Could you check a few things on this model? Use its own coordinates, in mm. Give positions to 0.01 mm unless a question says otherwise; leave off trailing zeros. Write each loop counter-clockwise with the first axis right and the second up, starting at its lowest first coordinate (ties: lowest second). Pieces come first, ordered by that corner, then holes. Notation, with made-up numbers: (73.5, 54) - (96.5, 54) arc R20 cw to (96.5, 74) - close; hole circle Ø2 at (34.25, -1). An arc over 180 degrees is marked (long way). Use one line per item in the form item = value.
```python
from build123d import *

# Parameters (mm, degrees)
F0_R     = 2.0193
F0_R_2   = 14.2875
F0_R_3   = 2.5527
F0_R_4   = 2.8575
F1_DEPTH = 6.35


with BuildPart() as f1:
    # F0 (on Front) → F1 (new body)
    with BuildSketch(Plane.XZ):
        with BuildLine():
            ThreePointArc((-49.323942, 42.948766), (-63.830824, 30.807895), (-82.659198, 28.979589))
            ThreePointArc((-82.659198, 28.979589), (-86.073502, 27.415326), (-85.607225, 23.688803))
            Line((-85.607225, 23.688803), (-45.021703, -19.243367))
            ThreePointArc((-45.021703, -19.243367), (-41.868292, -21.447891), (-38.1, -22.225))
            Line((-38.1, -22.225), (38.1, -22.225))
            ThreePointArc((38.1, -22.225), (41.868292, -21.447891), (45.021703, -19.243367))
            Line((45.021703, -19.243367), (85.607225, 23.688803))
            ThreePointArc((85.607225, 23.688803), (86.073502, 27.415326), (82.659198, 28.979589))
            ThreePointArc((82.659198, 28.979589), (63.830824, 30.807895), (49.323942, 42.948766))
            Line((49.323942, 42.948766), (22.663343, 84.185078))
            ThreePointArc((22.663343, 84.185078), (0, 96.52), (-22.663343, 84.185078))
            Line((-22.663343, 84.185078), (-49.323942, 42.948766))
        make_face()
        with Locations((-53.975, -1.5875)):
            Circle(F0_R, mode=Mode.SUBTRACT)
        with Locations((-38.1, -12.7)):
            Circle(F0_R, mode=Mode.SUBTRACT)
        with Locations((-38.1, 0)):
            Circle(F0_R, mode=Mode.SUBTRACT)
        with Locations((0, -1.5875)):
            Circle(F0_R_2, mode=Mode.SUBTRACT)
        with Locations((-38.1, 12.7)):
            Circle(F0_R, mode=Mode.SUBTRACT)
        with Locations((-31.75, 31.4325)):
            Circle(F0_R_3, mode=Mode.SUBTRACT)
        with Locations((38.1, -12.7)):
            Circle(F0_R, mode=Mode.SUBTRACT)
        with Locations((38.1, 0)):
            Circle(F0_R, mode=Mode.SUBTRACT)
        with Locations((53.975, -1.5875)):
            Circle(F0_R, mode=Mode.SUBTRACT)
        with Locations((38.1, 12.7)):
            Circle(F0_R, mode=Mode.SUBTRACT)
        with Locations((31.75, 31.4325)):
            Circle(F0_R_3, mode=Mode.SUBTRACT)
        with Locations((-25.4, 69.5325)):
            Circle(F0_R_4, mode=Mode.SUBTRACT)
        with Locations((0, 69.5325)):
            Circle(F0_R_2, mode=Mode.SUBTRACT)
        with Locations((25.4, 69.5325)):
            Circle(F0_R_4, mode=Mode.SUBTRACT)
    extrude(amount=F1_DEPTH)


solid = f1.part
```
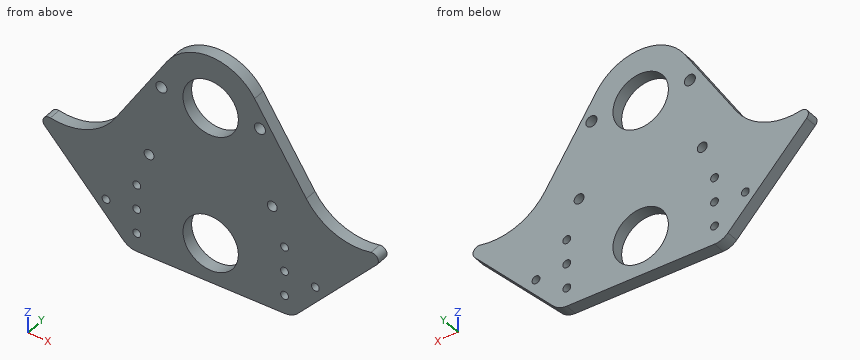
1. Imagine slicing it at D-D, the plane z = -12.7. List the corners of the cut face in (x, y) for me.
Response values:
outline = (-51.21, -6.35) - (-40.12, -6.35) - (-40.12, 0) - (-51.21, 0) - close; (-36.08, -6.35) - (-8.98, -6.35) - (-8.98, 0) - (-36.08, 0) - close; (8.98, -6.35) - (36.08, -6.35) - (36.08, 0) - (8.98, 0) - close; (40.12, -6.35) - (51.21, -6.35) - (51.21, 0) - (40.12, 0) - close
2. Imagine slicing it at B-B, the plane z = 79. List the corners of the cut face in (x, y) for me, and give its area (3 significant figures).
Response values:
outline = (-26.02, -6.35) - (-10.7, -6.35) - (-10.7, 0) - (-26.02, 0) - close; (10.7, -6.35) - (26.02, -6.35) - (26.02, 0) - (10.7, 0) - close
area = 195 mm²
3. Imagine slicing it at A-A, the plane x = 31.75. List the corners of the cut face in (y, z) for me (3 decimals), and give its area (3 significant figures).
Response values:
outline = (-6.35, -22.225) - (0, -22.225) - (0, 28.88) - (-6.35, 28.88) - close; (-6.35, 33.985) - (0, 33.985) - (0, 70.131) - (-6.35, 70.131) - close
area = 554 mm²
4. For pin 1 (4.5 mm diameter, centred on x = -25.4, z = 69.53, fed in from +Y); pin 2 (1 mm diameter, centred on x = -5, y = -1, fed in from +Z); pin 3 (2 mm diameter, centred on y = -4.5, z = -6.5, fed in from +X); pin 4 (1.5 mm diameter, centred on x = 61, y = -3.5, fed in from -Z), each with a flat end and sliding along its axis, tell me the tip position at first contact or that it passes through.
Response values:
pin_1 = through
pin_2 = 96.14
pin_3 = 58.01
pin_4 = -3.13
5. If I drill on line 1 (Z direction, x = 0, y = -4) (3 decimals); line 2 (X direction, y = -5, z = -1); line 3 (Z direction, x = 38.1, y = -4) (3 decimals), over which ranges is the centre line in solid material (lowest first)? Write a range as from..to.
Response values:
line_1 = -22.225..-15.875, 12.7..55.245, 83.82..96.52
line_2 = -62.27..-55.91, -52.04..-39.85, -36.35..-14.28, 14.28..36.35, 39.85..52.04, 55.91..62.27
line_3 = -22.225..-14.719, -10.681..-2.019, 2.019..10.681, 14.719..60.309
6. Imagine slicing it at C-C, the plane x = -11.5. List the corners of the cut face in (y, z) for me (3 decimals).
Response values:
outline = (-6.35, -22.225) - (0, -22.225) - (0, -10.066) - (-6.35, -10.066) - close; (-6.35, 6.891) - (0, 6.891) - (0, 61.054) - (-6.35, 61.054) - close; (-6.35, 78.011) - (0, 78.011) - (0, 93.947) - (-6.35, 93.947) - close
